from build123d import *

# Parameters (mm, degrees)
ESQUISSE1_W        = 300
ESQUISSE1_H        = 300
ESQUISSE1_W_2      = 275
ESQUISSE1_H_2      = 275
BOSS_EXTRU_1_DEPTH = 50
ESQUISSE2_W        = 275
ESQUISSE2_H        = 275
ESQUISSE2_W_2      = 245
ESQUISSE2_H_2      = 245
BOSS_EXTRU_2_DEPTH = 12
ESQUISSE3_W        = 25
ESQUISSE3_H        = 70
ESQUISSE3_W_2      = 70
ESQUISSE3_H_2      = 25
BOSS_EXTRU_3_DEPTH = 12


with BuildPart() as part:
    # Esquisse1 → Boss.-Extru.1 (new body)
    with BuildSketch(Plane.XY):
        Rectangle(ESQUISSE1_W, ESQUISSE1_H)
        Rectangle(ESQUISSE1_W_2, ESQUISSE1_H_2, mode=Mode.SUBTRACT)
    extrude(amount=BOSS_EXTRU_1_DEPTH)

    # Esquisse2 → Boss.-Extru.2 (add)
    with BuildSketch(Plane.XY):
        Rectangle(ESQUISSE2_W, ESQUISSE2_H)
        Rectangle(ESQUISSE2_W_2, ESQUISSE2_H_2, mode=Mode.SUBTRACT)
    extrude(amount=BOSS_EXTRU_2_DEPTH)

    # Esquisse3 → Boss.-Extru.3 (add)
    with BuildSketch(Plane.XY):
        with Locations((-0.890165861, 185)):
            Rectangle(ESQUISSE3_W, ESQUISSE3_H)
        with Locations((185, 0)):
            Rectangle(ESQUISSE3_W_2, ESQUISSE3_H_2)
        with Locations((-185, 0)):
            Rectangle(ESQUISSE3_W_2, ESQUISSE3_H_2)
        with Locations((-0.890165861, -185)):
            Rectangle(ESQUISSE3_W, ESQUISSE3_H)
    extrude(amount=BOSS_EXTRU_3_DEPTH)


solid = part.part
Source: CAD feature listing. Evaluate the final solid. Frame: model axes, mm. A direction names the side the tool comes from. Coordinates: 2 decimals unless noted, no trailing zeros. Loops run counter-clockwise (first coordinate to the right, second up) from the corner with the lowest first, then second, coordinate; pieces in that order, holes last. Notation, with made-up numbers: (43, 63.25) - (67, 63.25) arc R8 cw to (67, 71.25) - close; hole circle Ø3 at (51.5, 51). An arc over 180 degrees is marked (long way). One line per item, written item: value. Start each with the question number.
1. Ray query, L1, parallel to Y at x = 120, z = 46.5; L2, parallel to Y at x = 120, z = 8. Return the intervals inside material, ascending.
2. Mould query, pull axis Y, two halves, no side actions, for faces 1 (the flat face through (-185, -12.5, 6)), 2 (the flat face through (-137.5, -2, 31)), 3 (the flat face through (-1, 185, 12)). Classes: pulls with the +Y half, pulls with the -Y half, needs draft (parallel to the pull), parting line crosses it, or undercut.
3. Contact query for flat-ended pins moving along their axis: P1, Ø8, axis at y = -90.5, z = 25, coming from the +X side; P2, Ø8, axis at x = -171, z = 10, coming from the -Y side; P3, Ø3.5, axis at x = -189, z = 3.5, coming from the +Y side; P4, Ø8, axis at x = -121.5, y = -55, coming from the -Z side. Output: stop coordinate, or through.
4. Section D-D (z = 7). Return the cut outline in (x, y), and give its area (3 significant figures).
5. Section C-C (z = 43.5). Return the cut outline in (x, y), and give its area (3 significant figures).
6. Section A-A (x = 105). Return the cut outline in (y, z), and give its area (3 significant figures).
7. Set-up query: faces 4 (the flat face through (-2, -122.5, 6)), 5 (the flat face through (-1, -185, 12)), 6 (the flat face through (-13.39, -185, 6)), 7 (the flat face through (137.5, -2, 31)), 8 (the flat face through (185, -12.5, 6)). Return all of +Z, -Z, +X, -X, +Y, -Y with unobstructed straight access to the full face (end or side cutting, diameter ignored); none if empty.
Verdict:
1. L1: y = -150 to -137.5, 137.5 to 150
1. L2: y = -150 to -122.5, 122.5 to 150
2. face 1: pulls with the -Y half
2. face 2: undercut
2. face 3: needs draft
3. P1: stops at x = 150
3. P2: stops at y = -12.5
3. P3: stops at y = 12.5
3. P4: stops at z = 0
4. outline: (-220, -12.5) - (-150, -12.5) - (-150, -150) - (-13.39, -150) - (-13.39, -220) - (11.61, -220) - (11.61, -150) - (150, -150) - (150, -12.5) - (220, -12.5) - (220, 12.5) - (150, 12.5) - (150, 150) - (11.61, 150) - (11.61, 220) - (-13.39, 220) - (-13.39, 150) - (-150, 150) - (-150, 12.5) - (-220, 12.5) - close; hole (-122.5, -122.5) - (122.5, -122.5) - (122.5, 122.5) - (-122.5, 122.5) - close
4. area: 37,000 mm2
5. outline: (-150, -150) - (150, -150) - (150, 150) - (-150, 150) - close; hole (-137.5, -137.5) - (137.5, -137.5) - (137.5, 137.5) - (-137.5, 137.5) - close
5. area: 14,400 mm2
6. outline: (-150, 0) - (-122.5, 0) - (-122.5, 12) - (-137.5, 12) - (-137.5, 50) - (-150, 50) - close; (122.5, 0) - (150, 0) - (150, 50) - (137.5, 50) - (137.5, 12) - (122.5, 12) - close
6. area: 1,610 mm2
7. face 4: +Z, -Z
7. face 5: +Z, +X, -X, -Y
7. face 6: +Z, -Z, -X, -Y
7. face 7: +Z
7. face 8: +Z, -Z, +X, -Y
